Could you check a few things on this drawing? It's one solid part, dimensions in mm from its lowest x, y, z. Coordinates: 2 decimals unless noted, no trailing zeros. Order: outer loops, then holes, each group sorted by start corner. A loop starts at its lowest first (then second) coordinate and runs counter-clockwise, first axis right, second up. Notation, with made-up numbers: (81, -39.75) - (109, -39.75) arc R16 ccw to (109, -13.75) - close; hole circle Ø3 at (85.5, -11). An arc over 180 degrees is marked (long way). Return JSON: item names as keys, results as strings. Group by question number.
1) If I drill on line 1 along X through (y, z) = (24, 15.25); line 2 along X through (y, z) = (27, 12.5) (1 decimal); line 3 along Y through (x, z) = (16, 15) (1 decimal), over which ranges is the centre line in solid material (lowest first)?
2) Imagine slicing it at A-A (z = 16). Write out the boundary of the cut face in (x, y) (1 decimal).
3) For pin 1 Ø8 at (x, y) = (17.5, 22.5) entering from -Z (1 decimal), with a flat end and sliding along its axis, tell me the tip position at first contact or that it passes through.
4) If we mould it in two halves opening along Y, with no side actions, what happens to the marked faces 1, 2 and 3? For each: pulls with the +Y half, pulls with the -Y half, needs draft (parallel to the pull), parting line crosses it, or undercut.
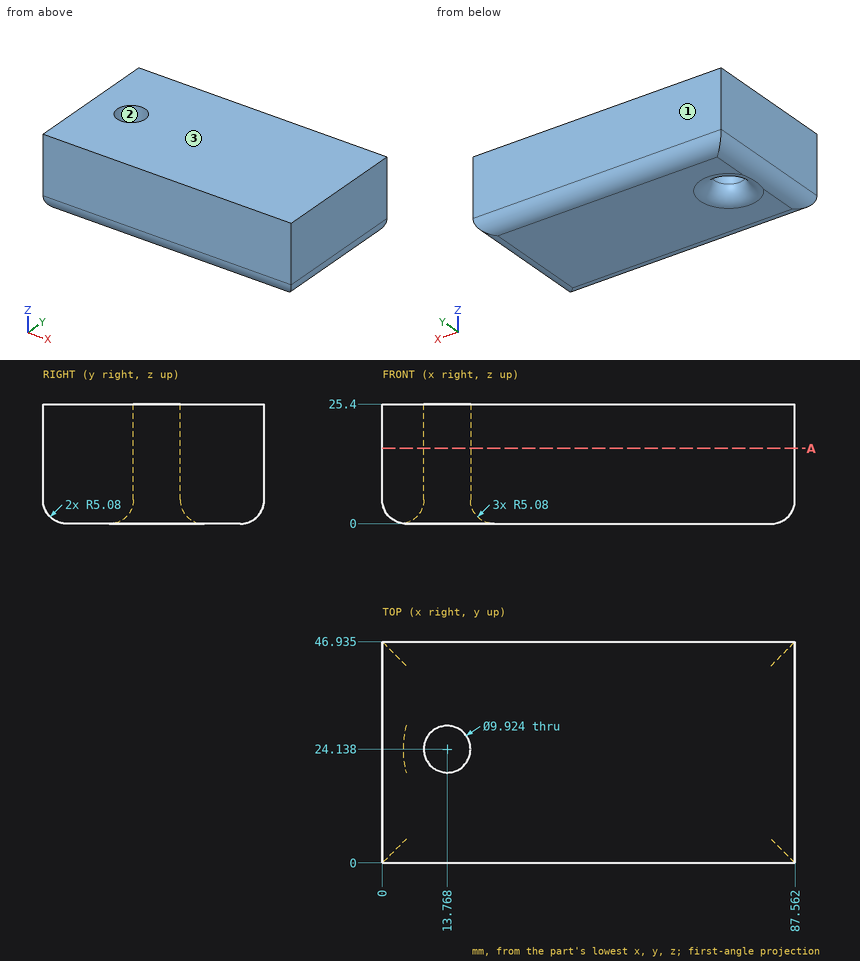
Calculated:
{
 "1": {"line 1": "0 to 8.81, 18.73 to 87.56", "line 2": "0 to 9.7, 17.8 to 87.6", "line 3": "0 to 19.7, 28.6 to 46.9"},
 "2": {"outline": "(0, 0) - (87.6, 0) - (87.6, 46.9) - (0, 46.9) - close; hole circle Ø9.9 at (13.8, 24.1)"},
 "3": {"pin 1": "z = 0.4"},
 "4": {"face 1": "pulls with the +Y half", "face 2": "undercut", "face 3": "needs draft"}
}
